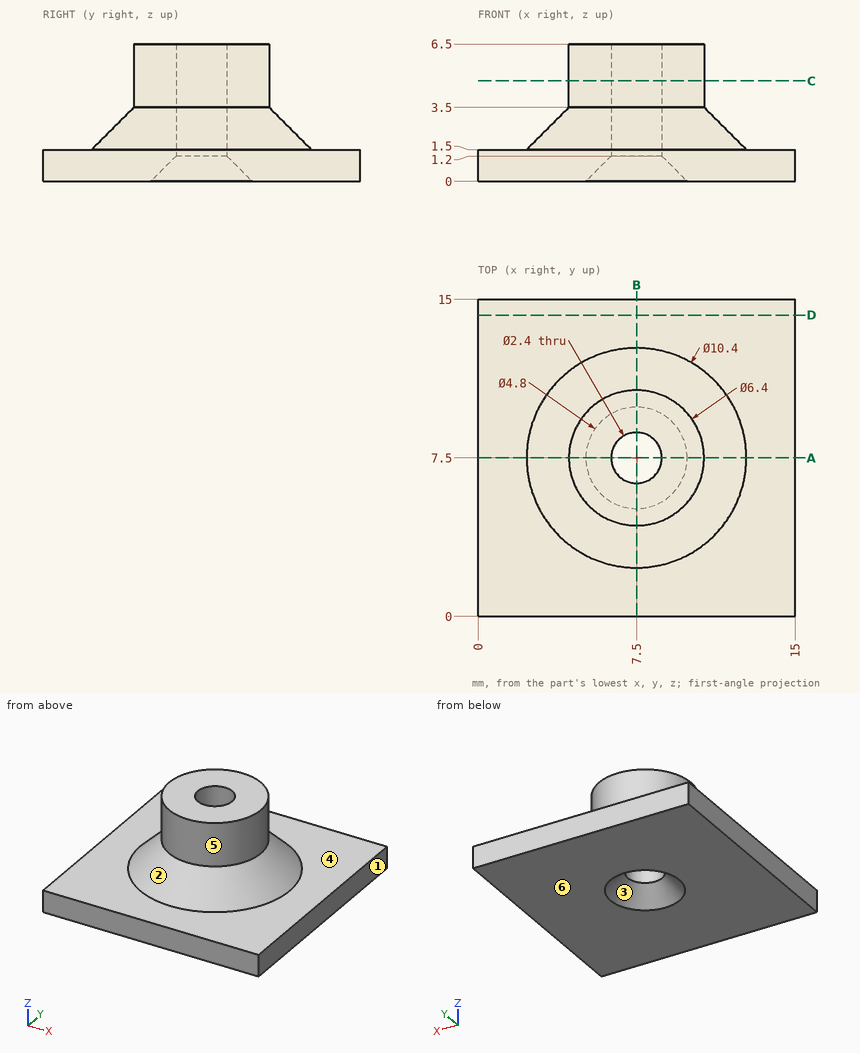
Check sheet for the drawn part. Datum: minimum x, y, z corner. Units: mm. A direction names the side the tool comes from. Coordinates: 2 decimals unless noted, no trailing zeros. Order: outer loops, then holes, each group sorted by start corner. A loop starts at its lowest first (then second) coordinate and runs counter-clockwise, first axis right, second up. Notation, with made-up numbers: (-5, -20) -> (31, -20) arc R14 ccw to (31, -4) -> close; hole circle Ø1 at (76, 31.5). An arc over 180 degrees is marked (long way). Use a Markdown table: item, result. Add a question column.
1. Mould release check, pull along X, two halves, no side actions. Record for the marked faces 1, 2, 3 and 4: pulls with the +X half, pulls with the -X half, needs draft (parallel to the pull), parting line crosses it, or undercut.
2. Material ranges on L1, parallel to Z at x = 0.5, y = 7; L2, parallel to X at y = 6.75, z = 6; L3, parallel to Y at x = 7.5, z = 3.3, recorded low to high.
3. Set-up check for the marked faces 5 and 6: record each of +Z, -Z, +X, -X, +Y, -Y from which the full face is reachable in a straight line by a thin tool's end or side.
4. Cross-section at C-C (z = 4.75). Enter the section's corners in (x, y).
5. Cross-section at D-D (y = 14.25). Enter the section's corners in (x, z).
6. Cross-section at A-A (y = 7.5). Enter the section's corners in (x, z), and give its area (3 significant figures).
7. Go/stop test with flat-tipped pins: pin 1 Ø1.5 at (y, z) = (7, 4.5) entering from -X; pin 2 Ø3 at (x, y) = (12, 9.5) entering from +Z. Record where each tip stops, or that it passes through.
Filled sheet:
| question | item | result |
|---|---|---|
| 1 | face 1 | pulls with the +X half |
| 1 | face 2 | parting line crosses it |
| 1 | face 3 | undercut |
| 1 | face 4 | needs draft |
| 2 | L1 | 0 to 1.5 |
| 2 | L2 | 4.39 to 6.56, 8.44 to 10.61 |
| 2 | L3 | 4.1 to 6.3, 8.7 to 10.9 |
| 3 | face 5 | +Z |
| 3 | face 6 | -Z, +X, -X, +Y, -Y |
| 4 | outline | circle Ø6.4 at (7.5, 7.5); hole circle Ø2.4 at (7.5, 7.5) |
| 5 | outline | (0, 0) -> (15, 0) -> (15, 1.5) -> (0, 1.5) -> close |
| 6 | outline | (0, 0) -> (5.1, 0) -> (6.3, 1.2) -> (6.3, 6.5) -> (4.3, 6.5) -> (4.3, 3.5) -> (2.3, 1.5) -> (0, 1.5) -> close; (8.7, 1.2) -> (9.9, 0) -> (15, 0) -> (15, 1.5) -> (12.7, 1.5) -> (10.7, 3.5) -> (10.7, 6.5) -> (8.7, 6.5) -> close |
| 6 | area | 41.5 mm2 |
| 7 | pin 1 | x = 4.3 |
| 7 | pin 2 | z = 3.28 |
